Read the model definition and answer for the solid it produces. Units are mm, in the model's axes. Face numbers are marked on the shaded views. A direction names the side the tool comes from. Round coordinates to 2 decimals unless told otherwise and drop trailing zeros. Order: outer loops, then holes, each group sorted by start corner. A loop starts at its lowest first (then second) coordinate and runs counter-clockwise, first axis right, second up. Notation, with made-up numbers: M 68.5,63.25 L 123.5,63.25 A7 cw 123.5,69.25 Z; hole C 75.25,-3 d5. An arc over 180 degrees is marked long. Use one line per item in the form item = value. Start each with the question number.
from build123d import *

# Parameters (mm, degrees)
F0_W      = 177.8
F0_H      = 177.8
F1_DEPTH  = 6.35
F2_W      = 19.7
F2_H      = 40.7
F3_DEPTH  = 20.5
F4_W      = 50.8
F4_H      = 76.2
F5_DEPTH  = 38.1
F6_W      = 74.8
F6_H      = 53
F7_DEPTH  = 6.35
F8_W      = 177.8
F8_H      = 6.35
F9_DEPTH  = 25.4
F10_W     = 16.9
F10_H     = 44.7
F11_DEPTH = 40
F13_D     = 5
F13_DEPTH = 12.7
F13_TIP   = 1.5021515476
F14_R     = 5.08


# Not quite as in the source:
# - a feature of the source that left no trace in its solid (it failed there, or was rolled back) is left out


with BuildPart() as f1:
    # F0 (on Top) → F1 (new body)
    with BuildSketch(Plane.XY):
        with Locations((-29.0734948754, -26.9331749929)):
            Rectangle(F0_W, F0_H)
    extrude(amount=F1_DEPTH)

    # F2 (on face) → F3 (join)
    with BuildSketch(Plane.XY.offset(6.35)):
        with Locations((49.9765051246, -37.5782008111)):
            Rectangle(F2_W, F2_H)
        with Locations((-108.1234948754, -37.5782008111)):
            Rectangle(F2_W, F2_H)
    extrude(amount=F3_DEPTH)

    # F4 (on face) → F5 (join)
    with BuildSketch(Plane.XY.offset(6.35)):
        with Locations((-25.4, -38.1)):
            Rectangle(F4_W, F4_H)
    extrude(amount=F5_DEPTH)

    # F6 (on face) → F7 (join)
    with BuildSketch(Plane.XY.offset(6.35)):
        with Locations((-10.0883172065, 34.7147134863)):
            Rectangle(F6_W, F6_H)
    extrude(amount=F7_DEPTH)

    # F8 (on face) → F9 (join)
    with BuildSketch(Plane.XY.offset(6.35)):
        with Locations((-29.0734948754, -112.6581749929)):
            Rectangle(F8_W, F8_H)
    extrude(amount=F9_DEPTH)

    # F10 (on face) → F11 (join)
    with BuildSketch(Plane.XY.offset(6.35)):
        with Locations((-78.1089827299, -87.1331749929)):
            Rectangle(F10_W, F10_H)
    extrude(amount=F11_DEPTH)

    # F13 (one way)
    with BuildSketch(Plane.YZ):
        with Locations((-58.6075335741, 23.0651237071), (-40.9188605845, 24.820599705), (-20.7475721836, 23.942861706)):
            Circle(F13_D / 2)
    extrude(amount=-F13_DEPTH, mode=Mode.SUBTRACT)
    with Locations(Plane.YZ):
        with Locations((-58.6075335741, 23.0651237071), (-40.9188605845, 24.820599705), (-20.7475721836, 23.942861706)):
            with Locations((0, 0, -(F13_DEPTH + F13_TIP / 2))):  # 118° drill point
                Cone(0, F13_D / 2, F13_TIP, mode=Mode.SUBTRACT)

    # F14
    f14_edges = [f1.edges().sort_by_distance(p)[0] for p in [
        (-69.658983, -87.133175, 46.35),
        (-78.108983, -64.783175, 46.35),
        (-86.558983, -87.133175, 46.35),
        (-78.108983, -109.483175, 46.35),
        (-86.558983, -64.783175, 26.35),
        (-69.658983, -64.783175, 26.35),
        (-69.658983, -109.483175, 39.05),
        (-86.558983, -109.483175, 39.05),
    ]]
    fillet(f14_edges, radius=F14_R)


solid = f1.part
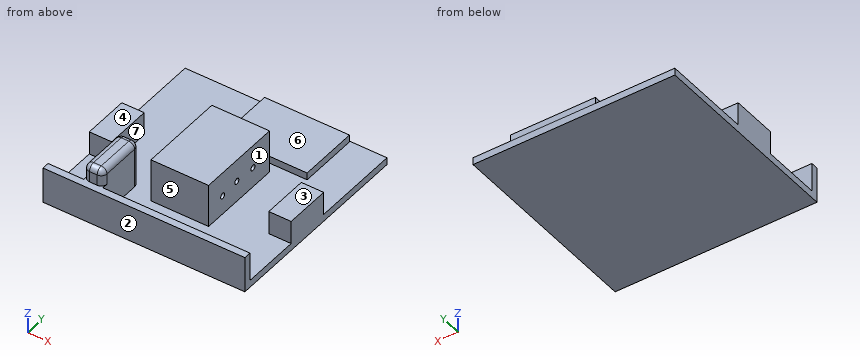
Item 1: Section D-D (y = -11) is taken. Write down the section's boundary in (x, z), and give its area (3 significant figures).
Item 2: Section B-B (z = 34.5) is taken. Write down the section's boundary in (x, y), and give its area (3 significant figures).
Item 3: A tool of negligible diameter and unlimited length cuts with its end or side. For the marked faces 4, 5, 6 and 7, from which of +Z, -Z, +X, -X, +Y, -Y can it reach the whole face along a straight path? Write none if from no direction.
Item 4: Section C-C (x = 48) is taken. Write down the section's boundary in (y, z), and give its area (3 significant figures).
Item 5: Section A-A (z = 9) is taken. Write down the section's boundary in (x, y), and give its area (3 significant figures).
Item 6: Given P1, Ø3.5, axis at x = -3, y = -108.5, coming from the +Z side; P2, Ø3, axis at y = -49, z = 41.5, coming from the -X side; P3, Ø6, axis at x = 47, z = 14, coming from the +Y side, each flat-ended and moving along its own axis, determine where each tip first touches the part or whether it passes through.
Item 7: For a pull along Y with two mould halves and no side action, classify the marked faces 1, 2 and 3 as pulls with the +Y half, pulls with the -Y half, needs draft (parallel to the pull), parting line crosses it, or undercut.
Item 8: Find the intervals of material crossed by L1, parallel to X at y = -22, z = 26.5; L2, parallel to Y at x = 46, z = 6.5; L3, parallel to Y at x = -18.5, z = 37, in increasing order. Write a range as [from, to].
The answers:
q1.outline = M -117.97,0 L 59.83,0 L 59.83,6.35 L 0,6.35 L 0,44.45 L -50.8,44.45 L -50.8,6.35 L -117.97,6.35 Z
q1.area = 3,060 mm²
q2.outline = M -86.56,-104.4 A5.08 ccw -81.48,-109.48 L -74.74,-109.48 A5.08 ccw -69.66,-104.4 L -69.66,-69.86 A5.08 ccw -74.74,-64.78 L -81.48,-64.78 A5.08 ccw -86.56,-69.86 Z; M -50.8,-76.2 L 0,-76.2 L 0,0 L -50.8,0 Z
q2.area = 4,600 mm²
q3.face_4 = +Z, -X, +Y
q3.face_5 = +Z, +X
q3.face_6 = +Z, +X, -X, +Y
q3.face_7 = +Z, +Y
q4.outline = M -115.83,0 L 61.97,0 L 61.97,6.35 L -17.23,6.35 L -17.23,26.85 L -57.93,26.85 L -57.93,6.35 L -109.48,6.35 L -109.48,31.75 L -115.83,31.75 Z
q4.area = 2,120 mm²
q5.outline = M -117.97,-115.83 L 59.83,-115.83 L 59.83,-109.48 L -69.66,-109.48 L -69.66,-69.86 A5.08 ccw -74.74,-64.78 L -81.48,-64.78 A5.08 ccw -86.56,-69.86 L -86.56,-109.48 L -117.97,-109.48 Z; M -117.97,-57.93 L -98.27,-57.93 L -98.27,-17.23 L -117.97,-17.23 Z; M -50.8,-76.2 L 0,-76.2 L 0,0 L -50.8,0 Z; M -47.49,8.21 L 27.31,8.21 L 27.31,61.21 L -47.49,61.21 Z; M 40.13,-57.93 L 59.83,-57.93 L 59.83,-17.23 L 40.13,-17.23 Z
q5.area = 11,300 mm²
q6.P1 = 31.75
q6.P2 = -50.8
q6.P3 = -17.23
q7.face_1 = undercut
q7.face_2 = pulls with the -Y half
q7.face_3 = needs draft
q8.L1 = [-117.97, -98.27], [-50.8, 0], [40.13, 59.83]
q8.L2 = [-115.83, -109.48], [-57.93, -17.23]
q8.L3 = [-76.2, 0]
